from build123d import *

# Parameters (mm, degrees)
F1_DEPTH = 25.4
F0_W     = 482.6
F0_H     = 50.8
F0_W_2   = 152.4
F2_W     = 2438.4
F2_H     = 50.8
F3_DEPTH = 25.4
F5_W     = 304.8
F5_H     = 50.8
F6_DEPTH = 63.5
F7_ANGLE = -90


with BuildPart() as f1:
    # F0 (on Top) → F1 (new body)
    with BuildSketch(Plane.XY):
        Polygon((-76.2, 0), (0, 0), (76.2, 0), (76.2, 50.8), (-76.2, 50.8), align=None)
    extrude(amount=F1_DEPTH)


with BuildPart() as f1b:
    # F0 (on Top) → F1, piece 2 (new body)
    with BuildSketch(Plane.XY):
        with Locations((-977.9, 25.4)):
            Rectangle(F0_W, F0_H)
    extrude(amount=F1_DEPTH)


with BuildPart() as f1c:
    # F0 (on Top) → F1, piece 3 (new body)
    with BuildSketch(Plane.XY):
        with Locations((977.9, 25.4)):
            Rectangle(F0_W, F0_H)
    extrude(amount=F1_DEPTH)


with BuildPart() as f1d:
    # F0 (on Top) → F1, piece 4 (new body)
    with BuildSketch(Plane.XY):
        with Locations((203.2, 25.4)):
            Rectangle(F0_W_2, F0_H)
    extrude(amount=F1_DEPTH)


with BuildPart() as f1e:
    # F0 (on Top) → F1, piece 5 (new body)
    with BuildSketch(Plane.XY):
        with Locations((406.4, 25.4)):
            Rectangle(F0_W_2, F0_H)
    extrude(amount=F1_DEPTH)


with BuildPart() as f1f:
    # F0 (on Top) → F1, piece 6 (new body)
    with BuildSketch(Plane.XY):
        with Locations((609.6, 25.4)):
            Rectangle(F0_W_2, F0_H)
    extrude(amount=F1_DEPTH)


with BuildPart() as f1g:
    # F0 (on Top) → F1, piece 7 (new body)
    with BuildSketch(Plane.XY):
        with Locations((-203.2, 25.4)):
            Rectangle(F0_W_2, F0_H)
    extrude(amount=F1_DEPTH)


with BuildPart() as f1h:
    # F0 (on Top) → F1, piece 8 (new body)
    with BuildSketch(Plane.XY):
        with Locations((-406.4, 25.4)):
            Rectangle(F0_W_2, F0_H)
    extrude(amount=F1_DEPTH)


with BuildPart() as f1i:
    # F0 (on Top) → F1, piece 9 (new body)
    with BuildSketch(Plane.XY):
        with Locations((-609.6, 25.4)):
            Rectangle(F0_W_2, F0_H)
    extrude(amount=F1_DEPTH)


with BuildPart() as f3:
    # F2 (on face) → F3 (new body)
    with BuildSketch(Plane.XY.offset(25.4)):
        with Locations((0, 25.4)):
            Rectangle(F2_W, F2_H)
    extrude(amount=F3_DEPTH)


with BuildPart() as f1b_1:
    add(f1b.part)

    # F4: union F1c, F1, F1d, F1e, F1f, F1g, F1h, F1i, F3
    add(f1c.part)
    add(f1.part)
    add(f1d.part)
    add(f1e.part)
    add(f1f.part)
    add(f1g.part)
    add(f1h.part)
    add(f1i.part)
    add(f3.part)

    # F5 (on face) → F6 (cut)
    with BuildSketch(Plane.XZ):
        with Locations((-1066.8, 25.4)):
            Rectangle(F5_W, F5_H)
        with Locations((1066.8, 25.4)):
            Rectangle(F5_W, F5_H)
    extrude(amount=-F6_DEPTH, mode=Mode.SUBTRACT)


with BuildPart() as f1b_2:
    # F7: moved
    add(f1b_1.part.rotate(Axis((0, 0, 50.8), (1, 0, 0)), F7_ANGLE))


solid = f1b_2.part
The model under review builds one solid part; all positions refer to its coordinate system, in mm. A direction names the side the tool comes from. Round coordinates to 2 decimals unless told otherwise and drop trailing zeros. Loops run counter-clockwise (first coordinate to the right, second up) from the corner with the lowest first, then second, coordinate; pieces in that order, holes last. Notation, with made-up numbers: M 76.5,-4 L 96.5,-4 A18 cw 96.5,25 Z; hole C -5,25.25 d1. An arc over 180 degrees is marked long. Answer as a JSON object with one key per item and string values.
Item 1: Tool access review of faces 4 (the face through (-508, -25.4, 25)), 5 (the face through (202, -50.8, 25)): name each direction out of +Z, -Z, +X, -X, +Y, -Y from which nothing blocks a thin tool from reaching the whole face with its end or side.
Check sheet entries:
{"face 4": "+Z, -Z, -Y", "face 5": "+Z, -Z, +X, -X, -Y"}
Item 2: We need section A-A, the plane y = -37.5. State how many separate pieces and enclosed holes the cut face has, and give its area (3 significant figures).
Check sheet entries:
{"separate pieces": "9", "enclosed holes": "0", "area": "72,300 mm2"}
Item 3: Clearance check with a flat-ended pin moving along its axis: P1, Ø15, axis at x = 720.5, z = 38, coming from the -Y side. State where the tip first meets the part, or that it passes through.
Check sheet entries:
{"P1": "y = -25.4"}
Item 4: The part is to be moulded in two halves that separate along X. For faces 1 (the face through (-914.4, -26, 26)), 2 (the face through (101, -25.4, 25)), 3 (the face through (-13, 0, 25)), say which applies: +X half, -X half, draft (parallel to the pull), parting line (faces both ways), or undercut.
Check sheet entries:
{"face 1": "-X half", "face 2": "undercut", "face 3": "draft"}
Item 5: We need section B-B, the plane x = -509. State the section outline as (y, z) points.
Check sheet entries:
{"outline": "M -25.4,0 L 0,0 L 0,50.8 L -25.4,50.8 Z"}
Item 6: For line 1 along Y through (x, z) = (-693, 28), list the stretches that pass through material, from the lowest coordinate up.
Check sheet entries:
{"line 1": "-25.4 to 0"}
